Geometry: final body of the model. Coordinates: model frame, mm. Face numbers are marked on the shaded views. Give positions to 0.01 mm unless a question says otherwise; leave off trailing zeros. Write each loop counter-clockwise with the first axis right and the second up, starting at its lowest first coordinate (ties: lowest second). Pieces come first, ordered by that corner, then holes. Notation, with made-up numbers: (68, -38) -> (117, -38) arc R19 ccw to (117, -1) -> close; hole circle Ø2 at (0, 45). An arc over 180 degrees is marked (long way). Answer as a JSON object with one key per item and string values.
from build123d import *

# Parameters (mm, degrees)
F0_R     = 36.5
F0_R_2   = 26.5
F1_DEPTH = 3
F0_R_3   = 10.5
F2_DEPTH = 10
F3_W     = 2
F3_H     = 6
F4_DEPTH = 25


with BuildPart() as f1:
    # F0 (on Top) → F1 (new body)
    with BuildSketch(Plane.XY):
        Circle(F0_R)
        Circle(F0_R_2, mode=Mode.SUBTRACT)
    extrude(amount=F1_DEPTH)

    # F0 (on Top) → F2 (join)
    with BuildSketch(Plane.XY):
        Circle(F0_R_2)
        Circle(F0_R_3, mode=Mode.SUBTRACT)
    extrude(amount=F2_DEPTH)

    # F3 (on Top) → F4 (cut)
    with BuildSketch(Plane.XY):
        with Locations((-20, 0)):
            Rectangle(F3_W, F3_H)
        with Locations((-14, 0)):
            Rectangle(F3_W, F3_H)
        with Locations((20, 0)):
            Rectangle(F3_W, F3_H)
        with Locations((14, 0)):
            Rectangle(F3_W, F3_H)
    extrude(amount=F4_DEPTH, mode=Mode.SUBTRACT)


solid = f1.part
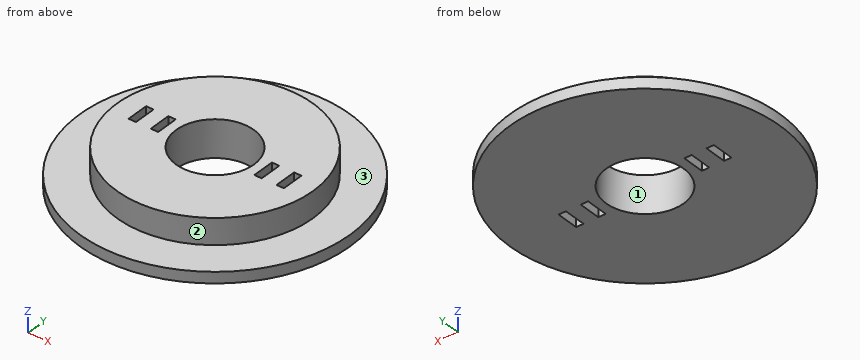
Q1. Cut plane A-A (y = 0). Return the cut outline in (x, z).
Values:
{"outline": "(-36.5, 0) -> (-21, 0) -> (-21, 10) -> (-26.5, 10) -> (-26.5, 3) -> (-36.5, 3) -> close; (-19, 0) -> (-15, 0) -> (-15, 10) -> (-19, 10) -> close; (-13, 0) -> (-10.5, 0) -> (-10.5, 10) -> (-13, 10) -> close; (10.5, 0) -> (13, 0) -> (13, 10) -> (10.5, 10) -> close; (15, 0) -> (19, 0) -> (19, 10) -> (15, 10) -> close; (21, 0) -> (36.5, 0) -> (36.5, 3) -> (26.5, 3) -> (26.5, 10) -> (21, 10) -> close"}
Q2. Mould query, pull axis Y, two halves, no side actions, for the marked faces 1, 2 and 3. Classes: pulls with the +Y half, pulls with the -Y half, needs draft (parallel to the pull), parting line crosses it, or undercut.
Values:
{"face 1": "undercut", "face 2": "parting line crosses it", "face 3": "needs draft"}
Q3. Cut plane C-C (z = 4.5). Return the cut outline in (x, y).
Values:
{"outline": "circle Ø53 at (0, 0); hole (-21, -3) -> (-19, -3) -> (-19, 3) -> (-21, 3) -> close; hole (-15, -3) -> (-13, -3) -> (-13, 3) -> (-15, 3) -> close; hole circle Ø21 at (0, 0); hole (13, -3) -> (15, -3) -> (15, 3) -> (13, 3) -> close; hole (19, -3) -> (21, -3) -> (21, 3) -> (19, 3) -> close"}
Q4. Cut plane D-D (y = -14.5). Return the cut outline in (x, z).
Values:
{"outline": "(-33.5, 0) -> (33.5, 0) -> (33.5, 3) -> (22.18, 3) -> (22.18, 10) -> (-22.18, 10) -> (-22.18, 3) -> (-33.5, 3) -> close"}
Q5. First-contact query: P1, Ø1.8, axis at y = -0.5, z = 3, coming from the -X side; P2, Ø2, axis at x = 20.5, z = 4.5, coming from the +Y side; P3, Ø1, axis at x = 19.5, z = 7, coming from the -Y side; P4, Ø5, axis at x = -9, z = 7, coming from the -Y side. Flat tips, straight axial feed; report the tip coordinate or a pass-through.
Values:
{"P1": "x = -36.5", "P2": "y = 17.94", "P3": "y = -18.47", "P4": "y = -25.69"}
Q6. Material intervals for L1, parallel to Y at x = 0.5, z = 1.75; L2, parallel to Z at x = -27, y = -1; L3, parallel to Y at x = 13.5, z = 7.5, sorted ascending. Write a range as from..to.
Values:
{"L1": "-36.5..-10.49, 10.49..36.5", "L2": "0..3", "L3": "-22.8..-3, 3..22.8"}
Q7. Cut plane B-B (x = 0). Return the cut outline in (y, z).
Values:
{"outline": "(-36.5, 0) -> (-10.5, 0) -> (-10.5, 10) -> (-26.5, 10) -> (-26.5, 3) -> (-36.5, 3) -> close; (10.5, 0) -> (36.5, 0) -> (36.5, 3) -> (26.5, 3) -> (26.5, 10) -> (10.5, 10) -> close"}
